Can you work these out from the model? Positions are in its coordinate system, mm. Coordinates: 2 decimals unless noted, no trailing zeros. Order: outer loops, then holes, each group sorted by start corner. A loop starts at its lowest first (then second) coordinate and runs counter-clockwise, first axis right, second up. Notation, with made-up numbers: (65, 65) - (107, 65) arc R29 cw to (107, 85) - close; hole circle Ø11 at (-39.5, 50.5). An arc over 180 degrees is marked (long way). Return JSON: item names as keys, results as strings. Group by question number.
1) Imagine slicing it at D-D (y = -6). Write out the boundary of the cut face in (x, z).
2) For pin 1 Ø6 at (y, z) = (-5, -11.5) entering from +X; pin 2 Ø6 at (y, z) = (-20, -0.5) entering from +X; pin 3 Ø12 at (y, z) = (-26, -21) entering from +X; pin 4 Ø3 at (x, y) = (-13.5, -12) entering from +Z, each with a flat end and sliding along its axis, tell me the tip position at first contact or that it passes through.
3) Imagine slicing it at B-B (x = 0). Write out the boundary of the cut face in (y, z), and give its area (3 significant figures).
4) Imagine slicing it at A-A (z = 0). Write out the boundary of the cut face in (x, y).
5) If we mould it in two halves opening along Y, with no side actions, what happens to faces 1 (the face through (0, -32, 0)), 2 (the face through (6, -10, 0)), 3 (the face through (-29.97, -4.97, 1.32)), 4 (the face through (0, 0, 0))? For each: pulls with the +Y half, pulls with the -Y half, needs draft (parallel to the pull), parting line crosses it, or undercut.
6) If I drill on line 1 along Y through (x, z) = (12.5, -16.5); line 2 along Z through (x, y) = (-0.5, -26.5); line 3 along Z through (x, y) = (-20, -6), over which ranges is the centre line in solid material (lowest first)?
7) Imagine slicing it at C-C (y = -20.5). Write out the boundary of the cut face in (x, z), and give its area (3 significant figures).
```python
from build123d import *

# Parameters (mm, degrees)
F0_R     = 30
F1_DEPTH = 10
F2_R     = 3
F3_R     = 5
F4_DEPTH = 6


with BuildPart() as f1:
    # F0 (on Front) → F1 (new body)
    with BuildSketch(Plane.XZ):
        Circle(F0_R)
    extrude(amount=F1_DEPTH)

    # F2
    f2_edges = [f1.edges().sort_by_distance(p)[0] for p in [
        (-30, -10, 0),
        (-30, 0, 0),
    ]]
    fillet(f2_edges, radius=F2_R)

    # F3 (on face) → F4 (join)
    with BuildSketch(Plane.XZ.offset(10)):
        Circle(F3_R)
    extrude(amount=F4_DEPTH)

    # F5: F1 across face


with BuildPart() as f1_1:
    add(f1.part)
    add(f1.part.mirror(Plane.XZ.offset(16)))


solid = f1_1.part
```
Calculated:
{
 "1": {"outline": "circle Ø60 at (0, 0)"},
 "2": {"pin 1": "x = 28.77", "pin 2": "x = 29.23", "pin 3": "x = 25.98", "pin 4": "through"},
 "3": {"outline": "(-32, -27) arc R3 ccw to (-29, -30) - (-25, -30) arc R3 ccw to (-22, -27) - (-22, -5) - (-10, -5) - (-10, -27) arc R3 ccw to (-7, -30) - (-3, -30) arc R3 ccw to (0, -27) - (0, 27) arc R3 ccw to (-3, 30) - (-7, 30) arc R3 ccw to (-10, 27) - (-10, 5) - (-22, 5) - (-22, 27) arc R3 ccw to (-25, 30) - (-29, 30) arc R3 ccw to (-32, 27) - close", "area": "1,300 mm2"},
 "4": {"outline": "(-30, -29) arc R3 ccw to (-27, -32) - (27, -32) arc R3 ccw to (30, -29) - (30, -25) arc R3 ccw to (27, -22) - (5, -22) - (5, -10) - (27, -10) arc R3 ccw to (30, -7) - (30, -3) arc R3 ccw to (27, 0) - (-27, 0) arc R3 ccw to (-30, -3) - (-30, -7) arc R3 ccw to (-27, -10) - (-5, -10) - (-5, -22) - (-27, -22) arc R3 ccw to (-30, -25) - close"},
 "5": {"face 1": "pulls with the -Y half", "face 2": "undercut", "face 3": "needs draft", "face 4": "pulls with the +Y half"},
 "6": {"line 1": "-32 to -22, -10 to 0", "line 2": "-30 to 30", "line 3": "-22.36 to 22.36"},
 "7": {"outline": "circle Ø10 at (0, 0)", "area": "78.5 mm2"}
}
